Part model, mm, in its own coordinate system. Face numbers are marked on the shaded views. Give positions to 0.01 mm unless a question says otherwise; leave off trailing zeros. Order: outer loops, then holes, each group sorted by start corner. A loop starts at its lowest first (then second) coordinate and runs counter-clockwise, first axis right, second up. Notation, with made-up numbers: (-27, 44) -> (8, 44) arc R16 ccw to (8, 56) -> close; hole circle Ø2 at (83.5, -2.75). An arc over 180 degrees is marked (long way). Write item = value, one per line. Start each with the question number.
(1) Probe line 1 along Z through (x, y) = (0, -0.65) (3 decimals); line 2 along Z through (x, y) = (20, -2.8); line 3 along Z through (x, y) = (-22.5, -2.65). List the from-to ranges inside material, lowest first. Write a range as from..to.
(2) Two-plate mould, pull along Y, no slides. Class the marked faces 1 and 2: pulls with the +Y half, pulls with the -Y half, needs draft (parallel to the pull), parting line crosses it, or undercut.
(3) Saw through at A-A, the plane z = 0. List the corners of the cut face in (x, y) (3 decimals).
(4) Saw through at B-B, the plane x = 0. List the corners of the cut face in (y, z) (3 decimals), then the cut area to 4 significant figures.
(5) Flat gauge pin, fed straight in: pin 1 (1.9 mm diameter, centred on x = 21.21, z = -21.21, fed in from +Y). Where does the tip first touch, or does it go through?
(6) Saw through at C-C, the plane y = -2.5. State how many separate pieces and enclosed holes the cut face has, then the cut area to 3 significant figures.
from build123d import *

# Parameters (mm, degrees)
F0_W     = 160
F0_H     = 80
F0_R     = 1.55
F0_R_2   = 2.5
F0_R_3   = 19.075
F1_DEPTH = 3


with BuildPart() as f1:
    # F0 (on Front) → F1 (new body)
    with BuildSketch(Plane.XZ):
        with Locations((-40, 0)):
            Rectangle(F0_W, F0_H)
        with Locations((-21.213203, -21.213203)):
            Circle(F0_R, mode=Mode.SUBTRACT)
        with Locations((0, -33.446151)):
            Circle(F0_R_2, mode=Mode.SUBTRACT)
        with Locations((21.213203, -21.213203)):
            Circle(F0_R, mode=Mode.SUBTRACT)
        with Locations((-33.446151, 0)):
            Circle(F0_R_2, mode=Mode.SUBTRACT)
        Circle(F0_R_3, mode=Mode.SUBTRACT)
        with Locations((33.446151, 0)):
            Circle(F0_R_2, mode=Mode.SUBTRACT)
        with Locations((-21.213203, 21.213203)):
            Circle(F0_R, mode=Mode.SUBTRACT)
        with Locations((21.213203, 21.213203)):
            Circle(F0_R, mode=Mode.SUBTRACT)
        with Locations((0, 33.446151)):
            Circle(F0_R_2, mode=Mode.SUBTRACT)
    extrude(amount=F1_DEPTH)


solid = f1.part
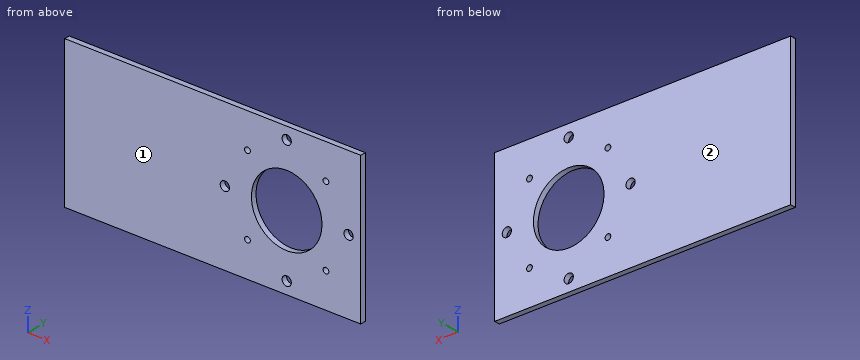
Results list:
q1.line_1 = -40..-35.946, -30.946..-19.075, 19.075..30.946, 35.946..40
q1.line_2 = -40..-22.18, -20.25..20.25, 22.18..40
q1.line_3 = -40..-22.08, -20.35..20.35, 22.08..40
q2.face_1 = pulls with the -Y half
q2.face_2 = pulls with the +Y half
q3.outline = (-120, -3) -> (-35.946, -3) -> (-35.946, 0) -> (-120, 0) -> close; (-30.946, -3) -> (-19.075, -3) -> (-19.075, 0) -> (-30.946, 0) -> close; (19.075, -3) -> (30.946, -3) -> (30.946, 0) -> (19.075, 0) -> close; (35.946, -3) -> (40, -3) -> (40, 0) -> (35.946, 0) -> close
q4.outline = (-3, -40) -> (0, -40) -> (0, -35.946) -> (-3, -35.946) -> close; (-3, -30.946) -> (0, -30.946) -> (0, -19.075) -> (-3, -19.075) -> close; (-3, 19.075) -> (0, 19.075) -> (0, 30.946) -> (-3, 30.946) -> close; (-3, 35.946) -> (0, 35.946) -> (0, 40) -> (-3, 40) -> close
q4.area = 95.55 mm^2
q5.pin_1 = through
q6.separate_pieces = 1
q6.enclosed_holes = 9
q6.area = 11,500 mm^2
